from build123d import *

# Parameters (mm, degrees)
BOSS_EXTRUDE1_DEPTH      = 1
BOSS_EXTRUDE2_DEPTH      = 11
BOSS_EXTRUDE3_DEPTH      = 5
BOSS_EXTRUDE3_DEPTH_BACK = 3
SKETCH3_W                = 50
SKETCH3_H                = 7
CUT_EXTRUDE3_DEPTH       = 25
SKETCH5_W                = 50
SKETCH5_H                = 7
CUT_EXTRUDE4_DEPTH       = 25
SKETCH6_W                = 50
SKETCH6_H                = 7
CUT_EXTRUDE5_DEPTH       = 25
SKETCH8_R                = 1.5
BOSS_EXTRUDE5_DEPTH      = 1
BOSS_EXTRUDE7_DEPTH      = 2.5


with BuildPart() as part:
    # Sketch1 → Boss-Extrude1 (new body)
    with BuildSketch(Plane(origin=(0, 0, 0), x_dir=(1, 0, 0), z_dir=(0, 1, 0))):
        Polygon((243.304219773, -116.484791866), (254.809280576, -136.408896139), (442.602090749, -136.409305398), (444.621046679, -132.925433223), (441.749040748, -132.925433223), (449.516726723, -119.471406457), (450.964695297, -121.978953122), (452.699916621, -118.984688017), (358.778179035, 43.666038066), (335.767496284, 43.666038066), align=None)
        Polygon((428.113670919, -116.417164681), (266.439108268, -116.428009241), (347.273609729, 23.609230825), align=None, mode=Mode.SUBTRACT)
    extrude(amount=BOSS_EXTRUDE1_DEPTH)

    # Sketch1_9 → Boss-Extrude2 (add)
    # profile 1 of 2: a face of its own
    with BuildSketch(Plane(origin=(0, 0, 0), x_dir=(1, 0, 0), z_dir=(0, 1, 0))):
        Polygon((229.159432547, -134.984249184), (231.716666588, -139.412373829), (462.829865412, -139.412373829), (465.38624875, -134.984588004), (349.829542096, 65.165499075), (344.716133219, 65.165499075), align=None)
        Polygon((251.922647988, -136.4093054), (233.446303399, -136.408896139), (232.623553959, -134.984217358), (241.860901688, -118.984688019), align=None, mode=Mode.SUBTRACT)
        Polygon((442.602090749, -136.409305398), (254.809280576, -136.408896139), (243.304219773, -116.484791866), (335.767496284, 43.666038066), (358.778179035, 43.666038066), (461.938967957, -134.984588004), (461.116393748, -136.409305398), align=None, mode=Mode.SUBTRACT)
        Polygon((348.096628302, 62.164013367), (357.334800991, 46.166038067), (337.210874326, 46.166038067), (346.44844193, 62.165948237), align=None, mode=Mode.SUBTRACT)
    # profile 2 of 2: a face of its own
    with BuildSketch(Plane(origin=(0, 0, 0), x_dir=(1, 0, 0), z_dir=(0, 1, 0))):
        Polygon((441.749040748, -132.925433223), (444.621046679, -132.925433223), (450.964695297, -121.978953122), (449.516726723, -119.471406457), align=None)
    extrude(amount=BOSS_EXTRUDE2_DEPTH)

    # Sketch1_10 → Boss-Extrude3 (add, two sides: drawn at the far end of the back side and taken through both)
    with BuildSketch(Plane(origin=(0, 0, 0), x_dir=(1, 0, 0), z_dir=(0, 1, 0)).offset(-BOSS_EXTRUDE3_DEPTH_BACK)):
        Polygon((229.159432547, -134.984249184), (231.716666588, -139.412373829), (462.829865412, -139.412373829), (465.38624875, -134.984588004), (349.829542096, 65.165499075), (344.716133219, 65.165499075), align=None)
        Polygon((251.922647988, -136.4093054), (233.446303399, -136.408896139), (232.623553959, -134.984217358), (241.860901688, -118.984688019), align=None, mode=Mode.SUBTRACT)
        Polygon((442.602090749, -136.409305398), (254.809280576, -136.408896139), (243.304219773, -116.484791866), (335.767496284, 43.666038066), (358.778179035, 43.666038066), (452.699916621, -118.984688017), (461.938967957, -134.984588004), (461.116393748, -136.409305398), align=None, mode=Mode.SUBTRACT)
        Polygon((348.096628302, 62.164013367), (357.334800991, 46.166038067), (337.210874326, 46.166038067), (346.44844193, 62.165948237), align=None, mode=Mode.SUBTRACT)
    extrude(amount=BOSS_EXTRUDE3_DEPTH + BOSS_EXTRUDE3_DEPTH_BACK)

    # Sketch3 → Cut-Extrude3 (cut)
    with BuildSketch(Plane(origin=(290.589645397, 0, -167.772009994), x_dir=(-0.49999999999998745, 0, -0.8660254037844459), z_dir=(0.8660254037844459, 0, -0.49999999999998745))):
        with Locations((-236.592990632, -3)):
            Rectangle(SKETCH3_W, SKETCH3_H)
    extrude(amount=-CUT_EXTRUDE3_DEPTH, mode=Mode.SUBTRACT)

    # Sketch5 → Cut-Extrude4 (cut)
    with BuildSketch(Plane.XY.offset(139.412373829)):
        with Locations((347.273266, -3)):
            Rectangle(SKETCH5_W, SKETCH5_H)
    extrude(amount=-CUT_EXTRUDE4_DEPTH, mode=Mode.SUBTRACT)

    # Sketch6 → Cut-Extrude5 (cut)
    with BuildSketch(Plane(origin=(230.319375797, 0, 132.975171838), x_dir=(-0.5000006154012504, 0, 0.8660250484820695), z_dir=(-0.8660250484820695, 0, -0.5000006154012504))):
        with Locations((-113.2366748, -3)):
            Rectangle(SKETCH6_W, SKETCH6_H)
    extrude(amount=-CUT_EXTRUDE5_DEPTH, mode=Mode.SUBTRACT)

    # Sketch8 → Boss-Extrude5 (add)
    with BuildSketch(Plane.XZ.offset(3)):
        Polygon((246.891774838, 127.696996709), (240.128710529, 115.984933576), (333.74677129, -46.166038067), (360.798886024, -46.166038067), (454.427535986, 116.00354071), (450.14703547, 123.280701064), (406.618322212, 98.678849058), (401.697951811, 107.384591709), (445.226665069, 131.986443715), (440.912417704, 139.412373829), (253.656752788, 139.412373829), align=None)
        with Locations(Location((395.323540807, 98.692824234, 0), (0, 0, 270))):
            Circle(SKETCH8_R, mode=Mode.SUBTRACT)
        with Locations(Location((348.301285092, 15.863526629, 0), (0, 0, 270))):
            Circle(SKETCH8_R, mode=Mode.SUBTRACT)
        with Locations(Location((299.654911442, 97.241681781, 0), (0, 0, 270))):
            Circle(SKETCH8_R, mode=Mode.SUBTRACT)
        Polygon((322.273266, 116.424264082), (294.358218631, 68.061097964), (319.354499366, 24.757680453), (376.473657317, 26.969372805), (401.47267951, 70.271207531), (372.273266, 116.420910258), align=None, mode=Mode.SUBTRACT)
    extrude(amount=BOSS_EXTRUDE5_DEPTH)

    # Sketch12 → Boss-Extrude7 (add)
    with BuildSketch(Plane(origin=(0, -3, 0), x_dir=(1, 0, 0), z_dir=(0, 1, 0))):
        with BuildLine():
            Line((347.505295142, -11.943526629), (347.306297654, -10.963526629))
            ThreePointArc((347.306297654, -10.963526629), (344.765751186, -12.327992723), (343.401285092, -14.868539192))
            Line((343.401285092, -14.868539192), (344.381285092, -15.067536679))
            ThreePointArc((344.381285092, -15.067536679), (345.472857967, -13.035099504), (347.505295142, -11.943526629))
        make_face()
        with BuildLine():
            ThreePointArc((353.201285092, -14.868539192), (351.836818997, -12.327992723), (349.296272529, -10.963526629))
            Line((349.296272529, -10.963526629), (349.097275041, -11.943526629))
            ThreePointArc((349.097275041, -11.943526629), (351.129712216, -13.035099504), (352.221285092, -15.067536679))
            Line((352.221285092, -15.067536679), (353.201285092, -14.868539192))
        make_face()
        with BuildLine():
            ThreePointArc((349.296272529, -20.763526629), (351.836818997, -19.399060535), (353.201285092, -16.858514066))
            Line((353.201285092, -16.858514066), (352.221285092, -16.659516578))
            ThreePointArc((352.221285092, -16.659516578), (351.129712216, -18.691953754), (349.097275041, -19.783526629))
            Line((349.097275041, -19.783526629), (349.296272529, -20.763526629))
        make_face()
        with BuildLine():
            Line((344.381285092, -16.659516578), (343.401285092, -16.858514066))
            ThreePointArc((343.401285092, -16.858514066), (344.765751186, -19.399060535), (347.306297654, -20.763526629))
            Line((347.306297654, -20.763526629), (347.505295142, -19.783526629))
            ThreePointArc((347.505295142, -19.783526629), (345.472857967, -18.691953754), (344.381285092, -16.659516578))
        make_face()
    extrude(amount=BOSS_EXTRUDE7_DEPTH)


solid = part.part
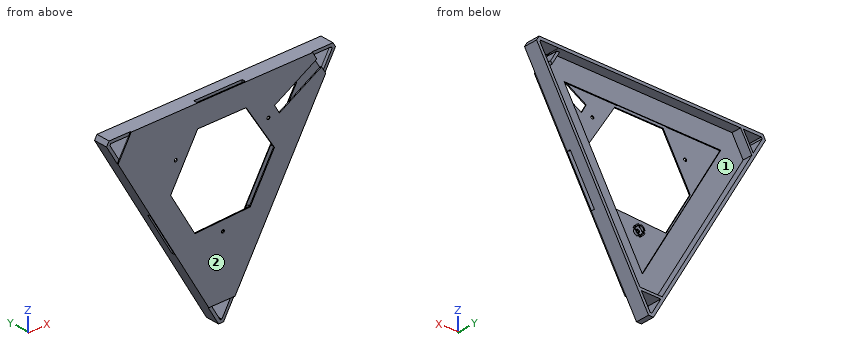
Part model, mm, in its own coordinate system. Face numbers are marked on the shaded views. Round coordinates to 2 decimals unless told otherwise and drop trailing zeros. Order: outer loops, then holes, each group sorted by start corner. A loop starts at its lowest first (then second) coordinate and runs counter-clockwise, first axis right, second up. Notation, with made-up numbers: (-16.75, -10) -> (35.25, -10) arc R24 cw to (35.25, 17) -> close; hole circle Ø6 at (42.5, 39.5). An arc over 180 degrees is marked (long way). Put each result on its own line as item: value.
Q1. Wall check: line 1 (Y direction, x = 428, z = 127); line 2 (Z direction, x = 408, y = 1.75); line 3 (X direction, y = 1.75, z = 106). Give the ranges that are in metal, low to high. Write a range as [from, to].
From the geometry:
line 1: y = [-4, -3], [0, 1]
line 2: z = [35.59, 41.57], [136.41, 139.41]
line 3: x = [245.89, 249.36], [445.2, 448.65]
Q2. Band-saw the part on D-D (x = 369). Give the cut face in (y, z), and give its area (3 significant figures).
From the geometry:
outline: (-4, -31.96) -> (11, -31.96) -> (11, -25.96) -> (1, -25.96) -> (1, 14.02) -> (0, 14.02) -> (0, -25.96) -> (-3, -25.96) -> (-3, 26.68) -> (-4, 26.68) -> close; (-4, 116.42) -> (-3, 116.42) -> (-3, 139.41) -> (-4, 139.41) -> close; (0.5, 116.42) -> (1, 116.42) -> (1, 136.41) -> (11, 136.41) -> (11, 139.41) -> (0.5, 139.41) -> close
area: 247 mm2
Q3. Band-saw the part on A-A (y = 5.5). Give the cut face in (x, z).
From the geometry:
outline: (229.16, 134.98) -> (344.72, -65.17) -> (349.83, -65.17) -> (465.39, 134.98) -> (462.83, 139.41) -> (231.72, 139.41) -> close; (441.75, 132.93) -> (449.52, 119.47) -> (450.96, 121.98) -> (444.62, 132.93) -> close; hole (232.62, 134.98) -> (241.86, 118.98) -> (251.92, 136.41) -> (233.45, 136.41) -> close; hole (243.3, 116.48) -> (335.77, -43.67) -> (358.78, -43.67) -> (461.94, 134.98) -> (461.12, 136.41) -> (442.6, 136.41) -> (254.81, 136.41) -> close; hole (337.21, -46.17) -> (346.45, -62.17) -> (348.1, -62.16) -> (357.33, -46.17) -> close
Q4. Pin check, flat tips, straight feed: pin 1 Ø2 at (y, z) = (0.5, 65) entering from -X; pin 2 Ø4.5 at (x, z) = (345, 18) entering from +Y; pin 3 Ø1 at (x, y) = (353, 4.5) entering from -Z; pin 4 Ø7 at (x, z) = (449.5, 124.5) entering from -Y. Stop position of each tip, or through.
From the geometry:
pin 1: stops at x = 268.99
pin 2: stops at y = -0.5
pin 3: stops at z = -60.54
pin 4: stops at y = -4
Q5. Pull direction X, two halves, no side cores. Call the marked faces 1 and 2: pulls with the +X half, pulls with the -X half, needs draft (parallel to the pull), parting line crosses it, or undercut.
From the geometry:
face 1: undercut
face 2: needs draft
Q6. Band-saw the part on C-C (x = 315). Give the cut face in (y, z), and give its area (3 significant figures).
From the geometry:
outline: (-4, -13.7) -> (11, -13.7) -> (11, -7.7) -> (1, -7.7) -> (1, 32.3) -> (0.5, 32.3) -> (0.5, 22.24) -> (0, 22.24) -> (0, -7.7) -> (-3, -7.7) -> (-3, 32.3) -> (-4, 32.3) -> close; (-4, 103.82) -> (-3, 103.82) -> (-3, 136.41) -> (0, 136.41) -> (0, 116.42) -> (1, 116.42) -> (1, 136.41) -> (11, 136.41) -> (11, 139.41) -> (-4, 139.41) -> close
area: 263 mm2
Q7. Band-saw the part on B-B (z = 43). Give the cut face in (x, y), and give its area (3 significant figures).
From the geometry:
outline: (282.27, -4) -> (308.82, -4) -> (308.82, -3) -> (282.27, -3) -> close; (282.27, 0.5) -> (308.82, 0.5) -> (308.82, 1) -> (285.73, 1) -> (285.73, 11) -> (282.27, 11) -> close; (385.73, -4) -> (412.28, -4) -> (412.28, -3) -> (385.73, -3) -> close; (385.73, 0.5) -> (412.28, 0.5) -> (412.28, 11) -> (408.82, 11) -> (408.82, 1) -> (385.73, 1) -> close
area: 149 mm2
